```python
from build123d import *

# Parameters (mm, degrees)
SKETCH1_W           = 60
SKETCH1_H           = 105
BOSS_EXTRUDE1_DEPTH = 4.4
SKETCH2_R           = 2.2
SKETCH2_R_2         = 6.7
SKETCH2_R_3         = 1.8
CUT_EXTRUDE1_DEPTH  = 61.626809251
CUT_EXTRUDE2_DEPTH  = 61.626809251
SKETCH5_R           = 8
SKETCH5_R_2         = 4.25
BOSS_EXTRUDE2_DEPTH = 4.3
CHAMFER1_SIZE       = 1
CUT_EXTRUDE3_DEPTH  = 61.626809251
BOSS_EXTRUDE3_START = 23.2
BOSS_EXTRUDE3_DEPTH = 23.2
SKETCH8_R           = 1.8
CUT_EXTRUDE4_DEPTH  = 67.468112656
FILLET1_R           = 10
BOSS_EXTRUDE4_DEPTH = 23.2
SKETCH11_R          = 1.8
CUT_EXTRUDE6_DEPTH  = 67.468112656
CUT_EXTRUDE5_DEPTH  = 23.6
CHAMFER2_SIZE       = 2


with BuildPart() as part:
    # Sketch1 → Boss-Extrude1 (new body)
    with BuildSketch(Plane(origin=(0, 0, 0), x_dir=(0, 0, -1), z_dir=(1, 0, 0))):
        Rectangle(SKETCH1_W, SKETCH1_H)
    extrude(amount=BOSS_EXTRUDE1_DEPTH)

    # Sketch2 → Cut-Extrude1 (cut, through all)
    with BuildSketch(Plane(origin=(4.4, 0, 0), x_dir=(0, 0, -1), z_dir=(1, 0, 0))):
        with Locations((0, 22.5)):
            Circle(SKETCH2_R)
        with Locations((0, -23.5)):
            Circle(SKETCH2_R_2)
        with Locations((-12.565, -23.5)):
            Circle(SKETCH2_R_3)
        with Locations((12.565, -23.5)):
            Circle(SKETCH2_R_3)
    extrude(amount=-CUT_EXTRUDE1_DEPTH, mode=Mode.SUBTRACT)

    # Sketch4 → Cut-Extrude2 (cut, through all)
    with BuildSketch(Plane(origin=(4.4, 0, 0), x_dir=(0, 0, -1), z_dir=(1, 0, 0))):
        with BuildLine():
            Line((-10.5, 8.55), (-0.5, 8.55))
            ThreePointArc((-0.5, 8.55), (1.25, 6.8), (-0.5, 5.05))
            Line((-0.5, 5.05), (-10.5, 5.05))
            ThreePointArc((-10.5, 5.05), (-12.25, 6.8), (-10.5, 8.55))
        make_face()
    extrude(amount=-CUT_EXTRUDE2_DEPTH, mode=Mode.SUBTRACT)

    # Sketch5 → Boss-Extrude2 (add)
    with BuildSketch(Plane.ZY):
        with Locations(Location((0, 22.5, 0), (0, 0, 180))):
            Circle(SKETCH5_R)
        with Locations(Location((0, 22.5, 0), (0, 0, 180))):
            Circle(SKETCH5_R_2, mode=Mode.SUBTRACT)
    extrude(amount=BOSS_EXTRUDE2_DEPTH)

    # Chamfer1
    chamfer1_edges = [part.edges().sort_by_distance(p)[0] for p in [
        (0, 22.5, 8),
    ]]
    chamfer(chamfer1_edges, length=CHAMFER1_SIZE)

    # Sketch6 → Cut-Extrude3 (cut, through all)
    with BuildSketch(Plane.ZY):
        with BuildLine():
            Line((-30, 52.5), (-30, 22.5))
            ThreePointArc((-30, 22.5), (-21.213203436, 43.713203436), (0, 52.5))
            Line((0, 52.5), (-30, 52.5))
        make_face()
        with BuildLine():
            Line((30, 52.5), (0, 52.5))
            ThreePointArc((0, 52.5), (21.213203436, 43.713203436), (30, 22.5))
            Line((30, 22.5), (30, 52.5))
        make_face()
    extrude(amount=-CUT_EXTRUDE3_DEPTH, mode=Mode.SUBTRACT)

    # Sketch7 → Boss-Extrude3 (add)
    with BuildSketch(Plane.ZY.offset(BOSS_EXTRUDE3_START)):
        with BuildLine():
            Line((-30, 22.5), (-30, 8))
            Line((-30, 8), (-27, 8))
            Line((-27, 8), (-25.4, 8))
            ThreePointArc((-25.4, 8), (-20.4, 13), (-25.4, 18))
            Line((-25.4, 18), (-27, 18))
            Line((-27, 18), (-27, 22.5))
            ThreePointArc((-27, 22.5), (0, 49.5), (27, 22.5))
            Line((27, 22.5), (27, 18))
            Line((27, 18), (25.4, 18))
            ThreePointArc((25.4, 18), (20.4, 13), (25.4, 8))
            Line((25.4, 8), (27, 8))
            Line((27, 8), (30, 8))
            Line((30, 8), (30, 22.5))
            ThreePointArc((30, 22.5), (0, 52.5), (-30, 22.5))
        make_face()
    extrude(amount=-BOSS_EXTRUDE3_DEPTH)

    # Sketch8 → Cut-Extrude4 (cut, through all)
    with BuildSketch(Plane.ZY.offset(23.2)):
        with Locations((-25.4, 13)):
            Circle(SKETCH8_R)
        with Locations((25.4, 13)):
            Circle(SKETCH8_R)
    extrude(amount=-CUT_EXTRUDE4_DEPTH, mode=Mode.SUBTRACT)

    # Fillet1
    fillet1_edges = [part.edges().sort_by_distance(p)[0] for p in [
        (2.2, -52.5, -30),
        (2.2, -52.5, 30),
    ]]
    fillet(fillet1_edges, radius=FILLET1_R)

    # Sketch10 → Boss-Extrude4 (add)
    with BuildSketch(Plane.ZY):
        with BuildLine():
            Line((20, -52.5), (-20, -52.5))
            ThreePointArc((-20, -52.5), (-27.071067812, -49.571067812), (-30, -42.5))
            Line((-30, -42.5), (-27, -42.5))
            ThreePointArc((-27, -42.5), (-19.464466094, -41.964466094), (-20, -49.5))
            Line((-20, -49.5), (20, -49.5))
            ThreePointArc((20, -49.5), (19.464466094, -41.964466094), (27, -42.5))
            Line((27, -42.5), (30, -42.5))
            ThreePointArc((30, -42.5), (27.071067812, -49.571067812), (20, -52.5))
        make_face()
    extrude(amount=BOSS_EXTRUDE4_DEPTH)

    # Sketch11 → Cut-Extrude6 (cut, through all)
    with BuildSketch(Plane.ZY.offset(23.2)):
        with Locations((-23, -45.5)):
            Circle(SKETCH11_R)
        with Locations((23, -45.5)):
            Circle(SKETCH11_R)
    extrude(amount=-CUT_EXTRUDE6_DEPTH, mode=Mode.SUBTRACT)

    # Sketch9 → Cut-Extrude5 (cut)
    with BuildSketch(Plane(origin=(4.4, 0, 0), x_dir=(0, 0, -1), z_dir=(1, 0, 0))):
        Polygon((-25.4, 9.709103466), (-22.55, 11.354551733), (-22.55, 14.645448267), (-25.4, 16.290896534), (-28.25, 14.645448267), (-28.25, 11.354551733), align=None)
        Polygon((25.4, 9.709103466), (28.25, 11.354551733), (28.25, 14.645448267), (25.4, 16.290896534), (22.55, 14.645448267), (22.55, 11.354551733), align=None)
        Polygon((-23, -42.209103466), (-25.85, -43.854551733), (-25.85, -47.145448267), (-23, -48.790896534), (-20.15, -47.145448267), (-20.15, -43.854551733), align=None)
        Polygon((23, -48.790896534), (25.85, -47.145448267), (25.85, -43.854551733), (23, -42.209103466), (20.15, -43.854551733), (20.15, -47.145448267), align=None)
    extrude(amount=-CUT_EXTRUDE5_DEPTH, mode=Mode.SUBTRACT)

    # Chamfer2
    # the kernel refuses this chamfer: 2 mm, written as the material it adds along each edge
    with BuildSketch(Plane(origin=(0, 12.856634024, -27), x_dir=(0.02749587661058639, 0, 0.9996219169112968), z_dir=(0, 1, 0))) as chamfer2_piece_1_section:
        Polygon((CHAMFER2_SIZE * 0.999621916911, -CHAMFER2_SIZE * 0.0274958766106), (-CHAMFER2_SIZE * 0.0274958766106, -CHAMFER2_SIZE * 0.999621916911), (0, 0), align=None)
    chamfer2_piece_1 = extrude(amount=9.643365976, mode=Mode.PRIVATE)
    chamfer2_piece_1 = split(chamfer2_piece_1, bisect_by=Plane(origin=(-0.079985343, 16.613435796, -25.958654389), z_dir=(0, 0.866025403784439, 0.4999999999999995)), keep=Keep.TOP, mode=Mode.PRIVATE)
    add(chamfer2_piece_1)
    with BuildSketch(Plane(origin=(0, 22.5, 27), x_dir=(0.02749587661058639, 0, -0.9996219169112968), z_dir=(0, -1, 0))) as chamfer2_piece_2_section:
        Polygon((CHAMFER2_SIZE * 0.999621916911, -CHAMFER2_SIZE * 0.0274958766106), (-CHAMFER2_SIZE * 0.0274958766106, -CHAMFER2_SIZE * 0.999621916911), (0, 0), align=None)
    chamfer2_piece_2 = extrude(amount=9.643365976, mode=Mode.PRIVATE)
    chamfer2_piece_2 = split(chamfer2_piece_2, bisect_by=Plane(origin=(-0.629221359, 16.946033943, 24.265268722), z_dir=(0, 0.8660254037844389, 0.4999999999999995)), keep=Keep.TOP, mode=Mode.PRIVATE)
    add(chamfer2_piece_2)
    with BuildSketch(Plane(origin=(0, 22.5, 0), x_dir=(0, 0, -1), z_dir=(0, -1, 0))) as chamfer2_piece_3:
        Polygon((27 - CHAMFER2_SIZE, 0), (27, -CHAMFER2_SIZE), (27, 0), align=None)
    revolve(axis=Axis((0, 22.5, 0), (1, 0, 0)), revolution_arc=180)
    with BuildSketch(Plane(origin=(0, 13, 25.4), x_dir=(0, 1, 0), z_dir=(0, 0, 1))) as chamfer2_piece_4:
        Polygon((5 + CHAMFER2_SIZE, 0), (5, CHAMFER2_SIZE), (5, 0), align=None)
    revolve(axis=Axis((0, 13, 25.4), (-1, 0, 0)), revolution_arc=180)
    with BuildSketch(Plane(origin=(0, 8, 25.4), x_dir=(0.027495876610586365, -0.9996219169112968, 0), z_dir=(0, 0, 1)), Plane(origin=(0, 8, -30), x_dir=(0.027495876610586365, -0.9996219169112968, 0), z_dir=(0, 0, 1))) as chamfer2_piece_5:
        Polygon((CHAMFER2_SIZE * 0.999621916911, -CHAMFER2_SIZE * 0.0274958766106), (-CHAMFER2_SIZE * 0.0274958766106, -CHAMFER2_SIZE * 0.999621916911), (0, 0), align=None)
    extrude(amount=4.6)
    with BuildSketch(Plane(origin=(0, 13, -25.4), x_dir=(0, -1, 0), z_dir=(0, 0, -1))) as chamfer2_piece_6:
        Polygon((5 + CHAMFER2_SIZE, 0), (5, CHAMFER2_SIZE), (5, 0), align=None)
    revolve(axis=Axis((0, 13, -25.4), (-1, 0, 0)), revolution_arc=180)
    with BuildSketch(Plane(origin=(0, -42.5, -30), x_dir=(0.02749587661058639, 0.9996219169112968, 0), z_dir=(0, 0, 1))) as chamfer2_piece_7_section:
        Polygon((CHAMFER2_SIZE * 0.999621916911, CHAMFER2_SIZE * 0.0274958766106), (-CHAMFER2_SIZE * 0.0274958766106, CHAMFER2_SIZE * 0.999621916911), (0, 0), align=None)
    chamfer2_piece_7 = extrude(amount=8.143365976, mode=Mode.PRIVATE)
    chamfer2_piece_7 = split(chamfer2_piece_7, bisect_by=Plane(origin=(-0.399536962, -44.995246479, -27.825741256), z_dir=(0, 0.8660254037844387, -0.4999999999999999)), keep=Keep.TOP, mode=Mode.PRIVATE)
    add(chamfer2_piece_7)
    with BuildSketch(Plane(origin=(0, -42.5, 21.856634024), x_dir=(0.02749587661058639, 0.9996219169112968, 0), z_dir=(0, 0, 1))) as chamfer2_piece_8_section:
        Polygon((CHAMFER2_SIZE * 0.999621916911, CHAMFER2_SIZE * 0.0274958766106), (-CHAMFER2_SIZE * 0.0274958766106, CHAMFER2_SIZE * 0.999621916911), (0, 0), align=None)
    chamfer2_piece_8 = extrude(amount=8.143365976, mode=Mode.PRIVATE)
    chamfer2_piece_8 = split(chamfer2_piece_8, bisect_by=Plane(origin=(-0.031503092, -41.384608505, 21.571932838), z_dir=(0, 0.8660254037844383, 0.5000000000000008)), keep=Keep.TOP, mode=Mode.PRIVATE)
    add(chamfer2_piece_8)
    with BuildSketch(Plane(origin=(0, -45.5, 23), x_dir=(0, -0.9259929219168064, 0.37754087005246884), z_dir=(0, 0.37754087005246884, 0.9259929219168064))) as chamfer2_piece_9_section:
        Polygon((5 + CHAMFER2_SIZE, 0), (5, -CHAMFER2_SIZE), (5, 0), align=None)
    chamfer2_piece_9 = revolve(axis=Axis((0, -45.5, 23), (1, 0, 0)), revolution_arc=314.36288287, mode=Mode.PRIVATE)
    chamfer2_piece_9 = chamfer2_piece_9 & Plane(origin=(-0.670588615, -42.5, 20), x_dir=(0, 0, 1), z_dir=(1, 0, 0)) * Cylinder(10, 28, mode=Mode.PRIVATE)
    add(chamfer2_piece_9)
    with BuildSketch(Plane(origin=(0, -45.5, -23), x_dir=(0, -0.3775408700524707, -0.9259929219168057), z_dir=(0, -0.9259929219168057, 0.3775408700524707))) as chamfer2_piece_10_section:
        Polygon((5 + CHAMFER2_SIZE, 0), (5, -CHAMFER2_SIZE), (5, 0), align=None)
    chamfer2_piece_10 = revolve(axis=Axis((0, -45.5, -23), (1, 0, 0)), revolution_arc=314.36288287, mode=Mode.PRIVATE)
    chamfer2_piece_10 = chamfer2_piece_10 & Plane(origin=(-0.979908178, -42.5, -20), x_dir=(0, -1, 0), z_dir=(1, 0, 0)) * Cylinder(10, 28, mode=Mode.PRIVATE)
    add(chamfer2_piece_10)
    with BuildSketch(Plane(origin=(0, -49.5, -25.143365976), x_dir=(0.02749587661058639, 0.9996219169112968, 0), z_dir=(0, 0, 1))) as chamfer2_piece_11_section:
        Polygon((CHAMFER2_SIZE * 0.999621916911, CHAMFER2_SIZE * 0.0274958766106), (-CHAMFER2_SIZE * 0.0274958766106, CHAMFER2_SIZE * 0.999621916911), (0, 0), align=None)
    chamfer2_piece_11 = extrude(amount=50.286731952, mode=Mode.PRIVATE)
    chamfer2_piece_11 = split(chamfer2_piece_11, bisect_by=Plane(origin=(-0.67159105, -38.844675798, 5.772640341), z_dir=(0, -0.8660254037844397, -0.4999999999999982)), keep=Keep.TOP, mode=Mode.PRIVATE)
    chamfer2_piece_11 = split(chamfer2_piece_11, bisect_by=Plane(origin=(-0.67159105, -38.844675769, -5.77264029), z_dir=(0, -0.8660254037844408, 0.4999999999999964)), keep=Keep.TOP, mode=Mode.PRIVATE)
    add(chamfer2_piece_11)
    with BuildSketch(Plane(origin=(0, 18, -25.4), x_dir=(0.02749587661058639, 0.9996219169112968, 0), z_dir=(0, 0, -1))) as chamfer2_piece_12_section:
        Polygon((CHAMFER2_SIZE * 0.999621916911, -CHAMFER2_SIZE * 0.0274958766106), (-CHAMFER2_SIZE * 0.0274958766106, -CHAMFER2_SIZE * 0.999621916911), (0, 0), align=None)
    chamfer2_piece_12 = extrude(amount=6.743365976, mode=Mode.PRIVATE)
    chamfer2_piece_12 = split(chamfer2_piece_12, bisect_by=Plane(origin=(-0.666666667, 18.666666667, -30), z_dir=(0, 0, 1)), keep=Keep.TOP, mode=Mode.PRIVATE)
    add(chamfer2_piece_12)
    with BuildSketch(Plane(origin=(0, 18, 27), x_dir=(0.02749587661058639, 0.9996219169112968, 0), z_dir=(0, 0, -1))) as chamfer2_piece_13:
        Polygon((CHAMFER2_SIZE * 0.999621916911, -CHAMFER2_SIZE * 0.0274958766106), (-CHAMFER2_SIZE * 0.0274958766106, -CHAMFER2_SIZE * 0.999621916911), (0, 0), align=None)
    extrude(amount=1.6)


solid = part.part
```
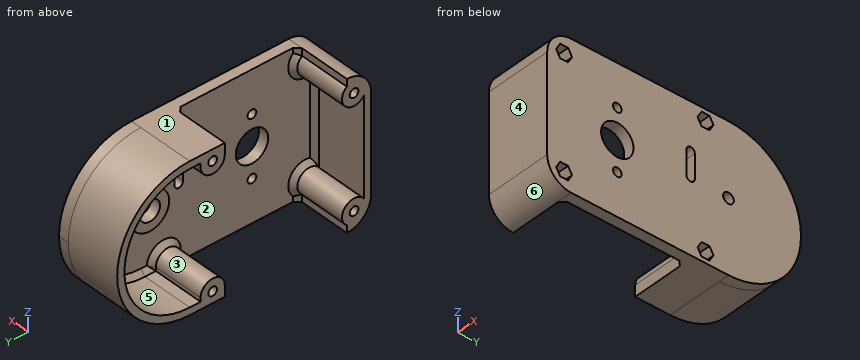
The model under review builds one solid part; all positions refer to its coordinate system, in mm. Face numbers are marked on the shaded views. A direction names the side the tool comes from. Give positions to 0.01 mm unless a question says otherwise; leave off trailing zeros. Write each loop counter-clockwise with the first axis right and the second up, starting at its lowest first coordinate (ties: lowest second). Pieces come first, ordered by that corner, then holes. Notation, with made-up numbers: (36, 82.25) -> (95, 82.25) arc R21 ccw to (95, 103.25) -> close; hole circle Ø5 at (-34, 72.5). An arc over 180 degrees is marked (long way). Put each result on its own line as item: value.
(1) The part is to be moulded in two halves that separate along Y. For the marked faces 1, 2, 3 and 4, say which applies: pulls with the +Y half, pulls with the -Y half, needs draft (parallel to the pull), parting line crosses it, or undercut.
Results are:
face 1: needs draft
face 2: undercut
face 3: undercut
face 4: pulls with the -Y half
(2) We need section B-B, the plane y = -23.5. Give the boundary of the cut face in (x, z) (3 decimals), and give its area (3 significant figures).
Results are:
outline: (0, -30) -> (4.4, -30) -> (4.4, -14.365) -> (0, -14.365) -> close; (0, -10.765) -> (4.4, -10.765) -> (4.4, -6.7) -> (0, -6.7) -> close; (0, 6.7) -> (4.4, 6.7) -> (4.4, 10.765) -> (0, 10.765) -> close; (0, 14.365) -> (4.4, 14.365) -> (4.4, 30) -> (0, 30) -> close
area: 173 mm²
(3) Tool access review of the marked faces 5 and 6: name each direction out of +Z, -Z, +X, -X, +Y, -Y from which nothing blocks a thin tool from reaching the whole face with its end or side.
Results are:
face 5: -X
face 6: -Z, +X, -X, -Y
(4) To check wall thickness, follow probe 1 along Y at (x, z) = (-17.5, 18.5); probe 2 along Z at (x, y) = (-5, 23); probe 3 along Y at (x, z) = (-22.05, -23). State the ranges of each line that lie inside material, in increasing order. Write a range as from..to.
Results are:
probe 1: -52.5..-49.5, -47.68..-43.32, 42.17..46.12
probe 2: -30..-27, 27..30
probe 3: -52.04..-47.3, -43.7..-40.5, 8.61..17.39, 36.64..41.76
(5) We need section C-C, the plane y = -45.5. Give the boundary of the cut face in (x, z), and give its area (3 significant figures).
Results are:
outline: (-23.2, -29.54) -> (4.4, -29.54) -> (4.4, -25.85) -> (-19.2, -25.85) -> (-19.2, -24.8) -> (-23.2, -24.8) -> close; (-23.2, -21.2) -> (-19.2, -21.2) -> (-19.2, -20.15) -> (4.4, -20.15) -> (4.4, 20.15) -> (-19.2, 20.15) -> (-19.2, 21.2) -> (-23.2, 21.2) -> (-23.2, 18) -> (-2, 18) -> (0, 16) -> (0, -16) -> (-2, -18) -> (-23.2, -18) -> close; (-23.2, 24.8) -> (-19.2, 24.8) -> (-19.2, 25.85) -> (4.4, 25.85) -> (4.4, 29.54) -> (-23.2, 29.54) -> close
area: 502 mm²
(6) We need section D-D, the plane x = -6.25. State how many separate pieces and enclosed holes the cut face has, and give its area (3 significant figures).
Results are:
separate pieces: 2
enclosed holes: 4
area: 674 mm²
(7) For pin 1 Ø2.5 at (x, z) = (-11.5, -29) entering from +Y; pin 2 Ø6 at (y, z) = (-14, 11) entering from -X; pin 3 Ø3 at (y, z) = (-45.5, -23) entering from +X; pin 4 Ø1 at (x, y) = (-12, -45.5) entering from +Z, all flat-tipped, find the tip position at first contact; note any pin that passes through.
Results are:
pin 1: y = 33.9
pin 2: x = 0
pin 3: through
pin 4: z = 29.68
(8) We need section A-A, the plane x = -21. Give the boundary of the cut face in (y, z).
Results are:
outline: (-52.5, -20) arc R10 ccw to (-42.5, -30) -> (-42.5, -27) arc R5 ccw (long way) to (-49.5, -20) -> (-49.5, 20) arc R5 ccw (long way) to (-42.5, 27) -> (-42.5, 30) arc R10 ccw to (-52.5, 20) -> close; (8, -30) -> (22.5, -30) arc R30 ccw to (22.5, 30) -> (8, 30) -> (8, 25.4) arc R5 ccw to (18, 25.4) -> (18, 27) -> (22.5, 27) arc R27 cw to (22.5, -27) -> (18, -27) -> (18, -25.4) arc R5 ccw to (8, -25.4) -> close; hole circle Ø3.6 at (-45.5, -23); hole circle Ø3.6 at (-45.5, 23); hole circle Ø3.6 at (13, -25.4); hole circle Ø3.6 at (13, 25.4)
